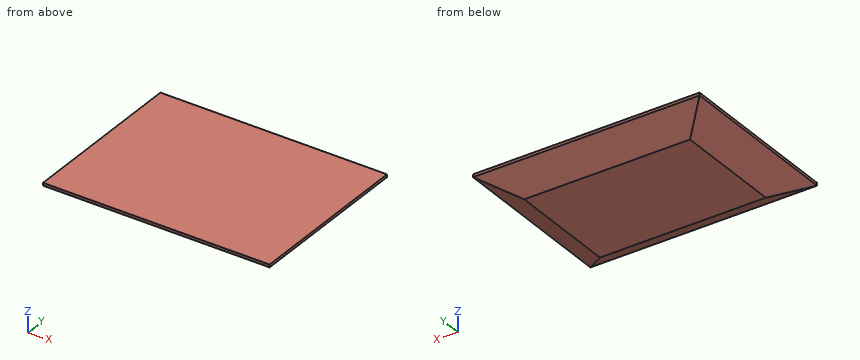
from build123d import *

# Parameters (mm, degrees)
F0_W     = 410
F0_H     = 310
F1_DEPTH = 35
F3_DEPTH = 413
F7_DEPTH = 455


with BuildPart() as f1:
    # F0 (on Top) → F1 (new body)
    with BuildSketch(Plane.XY):
        Rectangle(F0_W, F0_H)
    extrude(amount=F1_DEPTH)


with BuildPart() as f3:
    # F2 (on face) → F3 (new body)
    with BuildSketch(Plane.XZ.offset(155)):
        Polygon((-186.286226, -45.123053), (-150, 0), (-205, 30), (-247.468904, 11.412853), align=None)
    extrude(amount=-F3_DEPTH)


with BuildPart() as f4_1:
    # F4: instance of F3
    add(f3.part.mirror(Plane.YZ))


with BuildPart() as f1_1:
    add(f1.part)

    # F5: cut F3, F4_1
    add(f3.part, mode=Mode.SUBTRACT)
    add(f4_1.part, mode=Mode.SUBTRACT)


with BuildPart() as f7:
    # F6 (on face) → F7 (new body)
    with BuildSketch(Plane(origin=(-205, 0, 0), x_dir=(0, -1, 0), z_dir=(-1, 0, 0))):
        Polygon((-155, -27.468236), (-100, 0), (-155, 30), (-189.205855, 15.520646), align=None)
    extrude(amount=-F7_DEPTH)


with BuildPart() as f8_1:
    # F8: instance of F7
    add(f7.part.mirror(Plane.XZ))


with BuildPart() as f1_2:
    add(f1_1.part)

    # F9: cut F7, F8_1
    add(f7.part, mode=Mode.SUBTRACT)
    add(f8_1.part, mode=Mode.SUBTRACT)


solid = f1_2.part
Build history of the part. All positions in model axes, mm. Round coordinates to 2 decimals unless told otherwise and drop trailing zeros. Write each loop counter-clockwise with the first axis right and the second up, starting at its lowest first coordinate (ties: lowest second). Pieces come first, ordered by that corner, then holes. Notation, with made-up numbers: (-37.5, 51.5) - (-21.5, 51.5) arc R26 cw to (-21.5, 79.5) - close; hole circle Ø3 at (68.25, 38.5). An arc over 180 degrees is marked (long way). Use CSV: the item, a comma, the result in double quotes.
(1) Pin check, flat tips, straight feed: P1, Ø1, axis at x = -18.5, z = 24.5, coming from the -Y side; P2, Ø8, axis at x = -44, z = 25, coming from the -Y side; P3, Ø1, axis at x = -129.5, z = 14, coming from the -Y side. Stop position of each tip, or through.
Response:
P1,"y = -145.83"
P2,"y = -153.17"
P3,"y = -126.58"
(2) Band-saw the part on C-C (z = 15). Write the cut outline in (x, y).
Response:
outline,"(-177.5, -127.5) - (177.5, -127.5) - (177.5, 127.5) - (-177.5, 127.5) - close"
(3) Band-saw the part on A-A (x = -100.5). Write the cut outline in (y, z).
Response:
outline,"(-155, 30) - (-100, 0) - (100, 0) - (155, 30) - (155, 35) - (-155, 35) - close"
(4) Band-saw the part on B-B (y = -31.5). Write the cut outline in (x, z).
Response:
outline,"(-205, 30) - (-150, 0) - (150, 0) - (205, 30) - (205, 35) - (-205, 35) - close"
(5) Wall check: line 1 (Y direction, x = -26.5, z = 2.5); line 2 (X direction, y = -5, z = 23.5); line 3 (X direction, y = -33, z = 6). Give the ranges that are in metal, low to high.
Response:
line 1,"-104.58 to 104.58"
line 2,"-193.08 to 193.08"
line 3,"-161 to 161"
